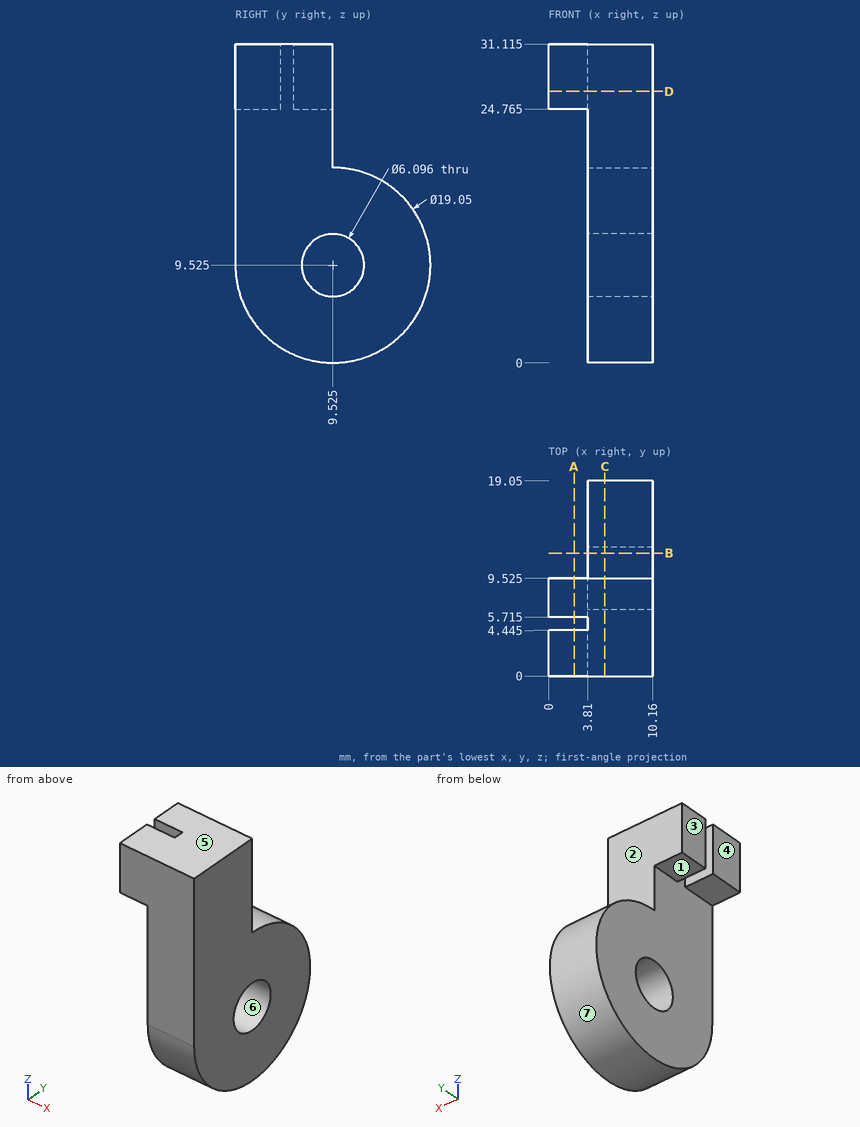
For this review, use the dimensioned drawing (mm, ordinates from the lowest corner) and the shaded views. A direction names the side the tool comes from. Give positions to 0.01 mm unless a question says otherwise; leave off trailing zeros. Loops run counter-clockwise (first coordinate to the right, second up) from the corner with the lowest first, then second, coordinate; pieces in that order, holes last.
Item 1: Take a section at C-C, the plane x = 5.5. State the section outline as (y, z) points (3 decimals), and give its area (3 significant figures).
Item 2: Tool access review of the marked faces 1, 2 and 3: name each direction out of +Z, -Z, +X, -X, +Y, -Y from which nothing blocks a thin tool from reaching the whole face with its end or side.
Item 3: For line 1 along X through (y, z) = (9, 3); line 2 along Z through (x, y) = (4.5, 10.5); line 3 along Y through (x, z) = (5.5, 24) (3 decimals), list the stretches that pass through material, from the lowest coordinate up.
Item 4: Take a section at B-B, the plane y = 12. State the section outline as (x, z) points, and give its area (3 significant figures).
Item 5: Draft analysis for pull direction Z (two halves, no side actions). For the marked faces 4, 5, 6 and 7, state which applies: +Z half, -Z half, draft (parallel to the pull), parting line (faces both ways), or undercut.
Item 6: Insertion check: pin 1 (5 mm diameter, centred on x = 8.5, y = 14.5, fed in from +Z); pin 2 (10 mm diameter, centred on y = 6, z = 9, fed in from -X); pin 3 (5 mm diameter, centred on x = 3.5, z = 26.5, fed in from +Y) (3 decimals). Each pin has a flat end and moves straight along its axis. Give the tip position at first contact, or say it passes through.
Item 7: Take a section at A-A, the plane x = 2.5. State the section outline as (y, z) points (3 decimals), and give its area (3 significant figures).
Item 8: Take a section at D-D, the plane z = 26.5. State the section outline as (x, y) points (3 decimals).
Calculated:
1. outline: (0, 9.525) arc R9.525 ccw (long way) to (9.525, 19.05) - (9.525, 31.115) - (0, 31.115) - close; hole circle Ø6.096 at (9.525, 9.525)
1. area: 390 mm2
2. face 1: -Z, -X, +Y, -Y
2. face 2: +Z, +X, -X, +Y
2. face 3: +Z, -Z, -X, +Y, -Y
3. line 1: x = 3.81 to 10.16
3. line 2: z = 0.05 to 6.64, 12.41 to 19
3. line 3: y = 0 to 9.525
4. outline: (3.81, 0.33) - (10.16, 0.33) - (10.16, 7.75) - (3.81, 7.75) - close; (3.81, 11.3) - (10.16, 11.3) - (10.16, 18.72) - (3.81, 18.72) - close
4. area: 94.2 mm2
5. face 4: draft
5. face 5: +Z half
5. face 6: undercut
5. face 7: parting line
6. pin 1: stops at z = 18.72
6. pin 2: stops at x = 3.81
6. pin 3: stops at y = 9.525
7. outline: (0, 24.765) - (4.445, 24.765) - (4.445, 31.115) - (0, 31.115) - close; (5.715, 24.765) - (9.525, 24.765) - (9.525, 31.115) - (5.715, 31.115) - close
7. area: 52.4 mm2
8. outline: (0, 0) - (10.16, 0) - (10.16, 9.525) - (0, 9.525) - (0, 5.715) - (3.81, 5.715) - (3.81, 4.445) - (0, 4.445) - close
